The listing builds one solid part. Answer for the finished solid, in the listing's coordinates (mm). A direction names the side the tool comes from. Coordinates: 2 decimals unless noted, no trailing zeros. Loops run counter-clockwise (first coordinate to the right, second up) from the corner with the lowest first, then second, coordinate; pieces in that order, holes last. Notation, with made-up numbers: (-33.75, 62) - (-16.75, 62) arc R31 cw to (-16.75, 97) - close; hole circle Ø2 at (-5, 67). An arc over 180 degrees is marked (long way). Return JSON: item names as keys, results as strings. Group by question number.
1. Which of the six approach directions +Z, -Z, +X, -X, +Y, -Y give full straight-line access (tool end or side, diameter ignored) to faces 1 (the face through (-7, -0.4, -1)), 2 (the face through (-10, 39.6, 1)), 3 (the face through (-14, 0, 1))?
2. Section A-A (y = 22) is taken. Write down the section's boundary in (x, z), and give its area (3 significant figures).
3. Find the intervals of material crossed by line 1 along Y through (x, z) = (-10.75, 2); line 2 along X through (y, z) = (20, -0.5); line 3 along Y through (x, z) = (-8.75, -3), in increasing order.
4. Each of these flat-tipped pins is pushed along its axis until it touches: P1, Ø8, axis at y = 19, z = -6.5, coming from the -X side; P2, Ø1, axis at x = -10, z = -1.5, coming from the +Y side; P3, Ø2, axis at x = -4.5, y = 9, coming from the -Z side; P4, Ø4, axis at x = -4, z = 4.5, coming from the -Y side. Where does it stop, or does it pass through?
```python
from build123d import *

# Parameters (mm, degrees)
SKETCH1_R            = 7.822299743
BOSS_EXTRUDE1_DEPTH  = 38.9
FILLET1_R            = 1
SKETCH7_R            = 6.058269956
BOSS_EXTRUDE7_DEPTH  = 0.7
FILLET5_R            = 1
SKETCH8_R            = 2.878199419
BOSS_EXTRUDE8_DEPTH  = 1.7
SKETCH9_R            = 1.57347679
BOSS_EXTRUDE9_DEPTH  = 0.7
FILLET7_R            = 0.5
SKETCH10_R           = 6.615584601
BOSS_EXTRUDE11_DEPTH = 0.2
FILLET8_R            = 0.5
FILLET9_R            = 0.5
SKETCH11_R           = 5.403530489
BOSS_EXTRUDE12_DEPTH = 0.2
FILLET10_R           = 0.5


with BuildPart() as part:
    # Sketch1 → Boss-Extrude1 (new body)
    with BuildSketch(Plane(origin=(0, 0, 0), x_dir=(1, 0, 0), z_dir=(0, 1, 0))):
        with Locations(Location((-7.367466469, 0.770235131, 0), (0, 0, 270))):
            Circle(SKETCH1_R)
    extrude(amount=BOSS_EXTRUDE1_DEPTH)

    # Fillet1
    fillet1_edges = [part.edges().sort_by_distance(p)[0] for p in [
        (-7.367466469, 38.9, -8.592534873),
    ]]
    fillet(fillet1_edges, radius=FILLET1_R)

    # Sketch7 → Boss-Extrude7 (add)
    with BuildSketch(Plane(origin=(0, 38.9, 0), x_dir=(1, 0, 0), z_dir=(0, 1, 0))):
        with Locations(Location((-7.367466469, 0.770235131, 0), (0, 0, 270))):
            Circle(SKETCH7_R)
    extrude(amount=BOSS_EXTRUDE7_DEPTH)

    # Fillet5
    # the kernel refuses this fillet: 1 mm, written as the material it takes off along each edge
    with BuildSketch(Plane(origin=(-7.367466469, 39.6, -0.770235131), x_dir=(0, 0, 1), z_dir=(-1, 0, 0))) as fillet5_piece_1:
        with BuildLine():
            CenterArc((5.104330755, -1), FILLET5_R, 17.457603124, 72.542396876)
            Line((5.104330755, 0), (5.104330755, 0.02))
            Line((5.104330755, 0.02), (6.058269956, 0.02))
            Line((6.058269956, 0.02), (6.078269956, 0))
            ThreePointArc((6.078269956, 0), (6.078269956, -0.35), (6.07734874, -0.694))
            Line((6.07734874, -0.694), (6.058269956, -0.7))
        make_face()
    revolve(axis=Axis((-7.367466469, 39.6, -0.770235131), (0, 1, 0)), mode=Mode.SUBTRACT)

    # Sketch8 → Boss-Extrude8 (add)
    with BuildSketch(Plane(origin=(0, 39.6, 0), x_dir=(1, 0, 0), z_dir=(0, 1, 0))):
        with Locations(Location((-7.367466469, 0.770235131, 0), (0, 0, 270))):
            Circle(SKETCH8_R)
    extrude(amount=BOSS_EXTRUDE8_DEPTH)

    # Sketch9 → Boss-Extrude9 (add)
    with BuildSketch(Plane(origin=(0, 41.3, 0), x_dir=(1, 0, 0), z_dir=(0, 1, 0))):
        with Locations(Location((-7.367466469, 0.770235131, 0), (0, 0, 270))):
            Circle(SKETCH9_R)
    extrude(amount=BOSS_EXTRUDE9_DEPTH)

    # Fillet7
    fillet7_edges = [part.edges().sort_by_distance(p)[0] for p in [
        (-7.367466469, 42, -2.343711921),
    ]]
    fillet(fillet7_edges, radius=FILLET7_R)

    # Sketch10 → Boss-Extrude11 (add)
    with BuildSketch(Plane.XZ):
        with Locations(Location((-7.367466469, -0.770235131, 0), (0, 0, 270))):
            Circle(SKETCH10_R)
    extrude(amount=BOSS_EXTRUDE11_DEPTH)

    # Fillet8
    fillet8_edges = [part.edges().sort_by_distance(p)[0] for p in [
        (-7.367466469, 0, -8.592534873),
    ]]
    fillet(fillet8_edges, radius=FILLET8_R)

    # Fillet9
    # the kernel refuses this fillet: 0.5 mm, written as the material it takes off along each edge
    with BuildSketch(Plane(origin=(-7.367466469, -0.2, -0.770235131), x_dir=(0, 0, -1), z_dir=(-1, 0, 0))) as fillet9_piece_1:
        with BuildLine():
            CenterArc((6.215584601, -0.5), FILLET9_R, 36.869897645, 53.130102355)
            Line((6.215584601, 0), (6.215584601, 0.01))
            Line((6.215584601, 0.01), (6.615584601, 0.01))
            Line((6.615584601, 0.01), (6.625584601, 0))
            ThreePointArc((6.625584601, 0), (6.625584601, -0.1), (6.623584601, -0.194))
            Line((6.623584601, -0.194), (6.615584601, -0.2))
        make_face()
    revolve(axis=Axis((-7.367466469, -0.2, -0.770235131), (0, -1, 0)), mode=Mode.SUBTRACT)

    # Sketch11 → Boss-Extrude12 (add)
    with BuildSketch(Plane.XZ.offset(0.2)):
        with Locations(Location((-7.367466469, -0.770235131, 0), (0, 0, 270))):
            Circle(SKETCH11_R)
    extrude(amount=BOSS_EXTRUDE12_DEPTH)

    # Fillet10
    # the kernel refuses this fillet: 0.5 mm, written as the material it takes off along each edge
    with BuildSketch(Plane(origin=(-7.367466469, -0.4, -0.770235131), x_dir=(0, 0, -1), z_dir=(-1, 0, 0))) as fillet10_piece_1:
        with BuildLine():
            CenterArc((5.003530489, -0.5), FILLET10_R, 36.869897645, 53.130102355)
            Line((5.003530489, 0), (5.003530489, 0.01))
            Line((5.003530489, 0.01), (5.403530489, 0.01))
            Line((5.403530489, 0.01), (5.413530489, 0))
            ThreePointArc((5.413530489, 0), (5.413530489, -0.1), (5.411530489, -0.194))
            Line((5.411530489, -0.194), (5.403530489, -0.2))
        make_face()
    revolve(axis=Axis((-7.367466469, -0.4, -0.770235131), (0, -1, 0)), mode=Mode.SUBTRACT)


solid = part.part
```
The answers:
{
 "1": {"face 1": "+Z, -Z, +X, -X, -Y", "face 2": "+Y", "face 3": "-Y"},
 "2": {"outline": "circle Ø15.64 at (-7.37, -0.77)", "area": "192 mm2"},
 "3": {"line 1": "y = -0.4 to 39.6", "line 2": "x = -15.19 to 0.45", "line 3": "y = -0.4 to 41.3"},
 "4": {"P1": "stops at x = -15", "P2": "stops at y = 41.3", "P3": "stops at z = -8.37", "P4": "stops at y = -0.4"}
}
